from build123d import *

# Parameters (mm, degrees)
SALIENTE_EXTRUIR1_DEPTH = 3
SKETCH1_W               = 20
SKETCH1_H               = 7
SKETCH1_H_2             = 8
SKETCH1_W_2             = 7
SKETCH1_H_3             = 38.5
BOSS_EXTRUDE1_DEPTH     = 23
CUT_EXTRUDE1_DEPTH      = 85.65548432
SKETCH3_R               = 1.625
CUT_EXTRUDE2_DEPTH      = 73.427902257
SKETCH4_R               = 1
CUT_EXTRUDE3_DEPTH      = 4
CORTAR_EXTRUIR1_DEPTH   = 10
CORTAR_EXTRUIR2_REACH   = 71.098
CROQUIS4_R              = 1.25
CORTAR_EXTRUIR3_DEPTH   = 3
BOSS_EXTRUDE2_DEPTH     = 20
SALIENTE_EXTRUIR2_DEPTH = 10
CORTAR_EXTRUIR4_REACH   = 91.44
CROQUIS7_R              = 1.625
CORTAR_EXTRUIR5_START   = -6.425484
CORTAR_EXTRUIR5_DEPTH   = 4
SALIENTE_EXTRUIR3_DEPTH = 10
CORTAR_EXTRUIR6_REACH   = 91.44
CROQUIS10_R             = 1.625
CORTAR_EXTRUIR7_START   = -2.42548
CORTAR_EXTRUIR7_DEPTH   = 4


with BuildPart() as part:
    # Croquis1 → Saliente-Extruir1 (new body)
    with BuildSketch(Plane(origin=(0, 0, 0), x_dir=(1, 0, 0), z_dir=(0, 1, 0))):
        Polygon((-29.5, 32.640625), (29.5, 32.640625), (29.5, -47.359375), (8.5, -47.359375), (8.5, -27.453125), (3.5, -27.453125), (3.5, -47.359375), (-3.5, -47.359375), (-3.5, -27.453125), (-8.5, -27.453125), (-8.5, -47.359375), (-29.5, -47.359375), align=None)
    extrude(amount=SALIENTE_EXTRUIR1_DEPTH)

    # Sketch1 → Boss-Extrude1 (add)
    with BuildSketch(Plane(origin=(0, 3, 0), x_dir=(1, 0, 0), z_dir=(0, 1, 0))):
        with Locations((0, 19.640625)):
            Rectangle(SKETCH1_W, SKETCH1_H)
        with Locations((0, -12.359375)):
            Rectangle(SKETCH1_W, SKETCH1_H_2)
        with Locations((0, -35.609375)):
            Rectangle(SKETCH1_W_2, SKETCH1_H_3)
    extrude(amount=BOSS_EXTRUDE1_DEPTH)

    # Sketch2 → Cut-Extrude1 (cut, through all)
    with BuildSketch(Plane(origin=(29.5, 0, 0), x_dir=(0, 0, -1), z_dir=(1, 0, 0))):
        Polygon((-54.859375, 26), (-46.359375, 0), (-47.359375, 0), (-47.359375, 3), (-54.859375, 3), align=None)
    extrude(amount=-CUT_EXTRUDE1_DEPTH, mode=Mode.SUBTRACT)

    # Sketch3 → Cut-Extrude2 (cut, through all)
    with BuildSketch(Plane.ZY.offset(10)):
        with Locations((12.359375, 5.75)):
            Circle(SKETCH3_R)
        with Locations((12.359375, 23.25)):
            Circle(SKETCH3_R)
    extrude(amount=-CUT_EXTRUDE2_DEPTH, mode=Mode.SUBTRACT)

    # Sketch4 → Cut-Extrude3 (cut)
    with BuildSketch(Plane(origin=(0, -13.692511694, 41.882976946), x_dir=(1, 0, 0), z_dir=(0, -0.31073885630742226, 0.9504953251756452))):
        with Locations(Location((0, 19.405659167, 0), (0, 0, 270))):
            Circle(SKETCH4_R)
        with Locations(Location((0, 29.405659167, 0), (0, 0, 270))):
            Circle(SKETCH4_R)
    extrude(amount=-CUT_EXTRUDE3_DEPTH, mode=Mode.SUBTRACT)

    # Croquis2 → Cortar-Extruir1 (cut)
    with BuildSketch(Plane(origin=(0, 0, -23.140625), x_dir=(-1, 0, 0), z_dir=(0, 0, -1))):
        Polygon((-5, 6), (-5, 3), (5, 3), (5, 6), (5, 21), (-5, 21), align=None)
    extrude(amount=-CORTAR_EXTRUIR1_DEPTH, mode=Mode.SUBTRACT)

    # Croquis3 → Cortar-Extruir2 (cut, up to next)
    with BuildSketch(Plane.ZY.offset(3.5), mode=Mode.PRIVATE) as cortar_extruir2_sk1:
        Polygon((21.90625, 3), (36.90625, 3), (36.90625, 26), (21.90625, 26), (16.359375, 26), (16.359375, 3), align=None)
    cortar_extruir2_tool1 = extrude(cortar_extruir2_sk1.sketch, amount=-CORTAR_EXTRUIR2_REACH, mode=Mode.PRIVATE) & part.part
    add(cortar_extruir2_tool1.solids().sort_by_distance((-3.5, 14.5, 26.632812))[0], mode=Mode.SUBTRACT)

    # Croquis4 → Cortar-Extruir3 (cut)
    with BuildSketch(Plane.XZ):
        with Locations(Location((-24.5, -22.640625, 0), (0, 0, 270))):
            Circle(CROQUIS4_R)
        with Locations(Location((-16.5, -22.640625, 0), (0, 0, 270))):
            Circle(CROQUIS4_R)
        with Locations(Location((-16.5, -12.640625, 0), (0, 0, 270))):
            Circle(CROQUIS4_R)
        with Locations(Location((-16.5, -2.640625, 0), (0, 0, 270))):
            Circle(CROQUIS4_R)
        with Locations(Location((-16.5, 7.359375, 0), (0, 0, 270))):
            Circle(CROQUIS4_R)
        with Locations(Location((-16.5, 17.359375, 0), (0, 0, 270))):
            Circle(CROQUIS4_R)
        with Locations(Location((-16.5, 27.359375, 0), (0, 0, 270))):
            Circle(CROQUIS4_R)
        with Locations(Location((-16.5, 37.359375, 0), (0, 0, 270))):
            Circle(CROQUIS4_R)
        with Locations(Location((-24.5, -12.640625, 0), (0, 0, 270))):
            Circle(CROQUIS4_R)
        with Locations(Location((-24.5, -2.640625, 0), (0, 0, 270))):
            Circle(CROQUIS4_R)
        with Locations(Location((-24.5, 7.359375, 0), (0, 0, 270))):
            Circle(CROQUIS4_R)
        with Locations(Location((-24.5, 17.359375, 0), (0, 0, 270))):
            Circle(CROQUIS4_R)
        with Locations(Location((-24.5, 27.359375, 0), (0, 0, 270))):
            Circle(CROQUIS4_R)
        with Locations(Location((-24.5, 37.359375, 0), (0, 0, 270))):
            Circle(CROQUIS4_R)
        with Locations(Location((16.5, 37.359375, 0), (0, 0, 270))):
            Circle(CROQUIS4_R)
        with Locations(Location((24.5, 37.359375, 0), (0, 0, 270))):
            Circle(CROQUIS4_R)
        with Locations(Location((16.5, 27.359375, 0), (0, 0, 270))):
            Circle(CROQUIS4_R)
        with Locations(Location((24.5, 27.359375, 0), (0, 0, 270))):
            Circle(CROQUIS4_R)
        with Locations(Location((16.5, 17.359375, 0), (0, 0, 270))):
            Circle(CROQUIS4_R)
        with Locations(Location((24.5, 17.359375, 0), (0, 0, 270))):
            Circle(CROQUIS4_R)
        with Locations(Location((24.5, 7.359375, 0), (0, 0, 270))):
            Circle(CROQUIS4_R)
        with Locations(Location((16.5, 7.359375, 0), (0, 0, 270))):
            Circle(CROQUIS4_R)
        with Locations(Location((16.5, -2.640625, 0), (0, 0, 270))):
            Circle(CROQUIS4_R)
        with Locations(Location((24.5, -2.640625, 0), (0, 0, 270))):
            Circle(CROQUIS4_R)
        with Locations(Location((24.5, -12.640625, 0), (0, 0, 270))):
            Circle(CROQUIS4_R)
        with Locations(Location((16.5, -12.640625, 0), (0, 0, 270))):
            Circle(CROQUIS4_R)
        with Locations(Location((16.5, -22.640625, 0), (0, 0, 270))):
            Circle(CROQUIS4_R)
        with Locations(Location((24.5, -22.640625, 0), (0, 0, 270))):
            Circle(CROQUIS4_R)
        with Locations(Location((6, 22.084531493, 0), (0, 0, 270))):
            Circle(CROQUIS4_R)
        with Locations(Location((-6, 22.084531493, 0), (0, 0, 270))):
            Circle(CROQUIS4_R)
        with Locations(Location((6, 2.359375, 0), (0, 0, 270))):
            Circle(CROQUIS4_R)
        with Locations(Location((-6, 2.359375, 0), (0, 0, 270))):
            Circle(CROQUIS4_R)
        with Locations(Location((-6, -7.640625, 0), (0, 0, 270))):
            Circle(CROQUIS4_R)
        with Locations(Location((6, -7.640625, 0), (0, 0, 270))):
            Circle(CROQUIS4_R)
    extrude(amount=-CORTAR_EXTRUIR3_DEPTH, mode=Mode.SUBTRACT)

    # Sketch5 → Boss-Extrude2 (add)
    with BuildSketch(Plane(origin=(-8.5, 0, 0), x_dir=(0, 0, -1), z_dir=(1, 0, 0))):
        Polygon((-36.90625, 3), (-36.90625, 0), (-46.359375, 0), (-47.340144231, 3), align=None)
    extrude(amount=BOSS_EXTRUDE2_DEPTH)

    # Croquis6 → Saliente-Extruir2 (add)
    with BuildSketch(Plane.ZY.offset(29.5)):
        Polygon((44.340144231, 3), (47.340144231, 3), (50.447532794, 12.504953252), (44.340144231, 14.501599513), (44.340144231, 6.347956044), align=None)
        Polygon((40.990144231, 3), (44.340144231, 3), (44.340144231, 6.347956044), align=None)
    extrude(amount=-SALIENTE_EXTRUIR2_DEPTH)

    # Cortar-Extruir4: up to this plane
    cortar_extruir4_end = Plane(origin=(-19.5, 0, 44.340144231), z_dir=(0, 0, -1))
    # Croquis7 → Cortar-Extruir4 (cut, up to the surface)
    with BuildSketch(Plane(origin=(0, -13.692511694, 41.882976946), x_dir=(1, 0, 0), z_dir=(0, -0.31073885630742226, 0.9504953251756452)), mode=Mode.PRIVATE) as cortar_extruir4_sk1:
        with Locations(Location((-24.5, 22.561908251, 0), (0, 0, 270))):
            Circle(CROQUIS7_R)
    cortar_extruir4_tool1 = split(extrude(cortar_extruir4_sk1.sketch, amount=-CORTAR_EXTRUIR4_REACH, mode=Mode.PRIVATE), bisect_by=cortar_extruir4_end, keep=Keep.BOTH, mode=Mode.PRIVATE)
    add(cortar_extruir4_tool1.solids().sort_by_distance((-24.5, 7.752477, 48.893839))[0], mode=Mode.SUBTRACT)

    # Croquis8 → Cortar-Extruir5 (cut)
    with BuildSketch(Plane(origin=(0, -13.692511694, 41.882976946), x_dir=(1, 0, 0), z_dir=(0, -0.31073885630742226, 0.9504953251756452)).offset(CORTAR_EXTRUIR5_START)):
        Polygon((-22.91228676, 19.811908251), (-21.324573519, 22.561908251), (-22.91228676, 25.311908251), (-26.08771324, 25.311908251), (-27.675426481, 22.561908251), (-26.08771324, 19.811908251), align=None)
    extrude(amount=CORTAR_EXTRUIR5_DEPTH, mode=Mode.SUBTRACT)

    # Croquis9 → Saliente-Extruir3 (add)
    with BuildSketch(Plane(origin=(29.5, 0, 0), x_dir=(0, 0, -1), z_dir=(1, 0, 0))):
        Polygon((-50.447532794, 12.504953252), (-47.340144231, 3), (-44.340144231, 3), (-44.340144231, 6.347956044), (-44.340144231, 14.501599513), align=None)
        Polygon((-44.340144231, 6.347956044), (-44.340144231, 3), (-40.990144231, 3), align=None)
    extrude(amount=-SALIENTE_EXTRUIR3_DEPTH)

    # Cortar-Extruir6: up to this plane
    cortar_extruir6_end = Plane(origin=(19.5, 0, 44.340144231), z_dir=(0, 0, 1))
    # Croquis10 → Cortar-Extruir6 (cut, up to the surface)
    with BuildSketch(Plane(origin=(0, -13.692511694, 41.882976946), x_dir=(1, 0, 0), z_dir=(0, -0.31073885630742226, 0.9504953251756452)), mode=Mode.PRIVATE) as cortar_extruir6_sk1:
        with Locations(Location((24.5, 22.561908251, 0), (0, 0, 270))):
            Circle(CROQUIS10_R)
    cortar_extruir6_tool1 = split(extrude(cortar_extruir6_sk1.sketch, amount=-CORTAR_EXTRUIR6_REACH, mode=Mode.PRIVATE), bisect_by=cortar_extruir6_end, keep=Keep.BOTH, mode=Mode.PRIVATE)
    add(cortar_extruir6_tool1.solids().sort_by_distance((24.5, 7.752477, 48.893839))[0], mode=Mode.SUBTRACT)

    # Croquis11 → Cortar-Extruir7 (cut)
    with BuildSketch(Plane(origin=(0, -13.692511694, 41.882976946), x_dir=(1, 0, 0), z_dir=(0, -0.31073885630742226, 0.9504953251756452)).offset(CORTAR_EXTRUIR7_START)):
        Polygon((26.08771324, 19.811908251), (27.675426481, 22.561908251), (26.08771324, 25.311908251), (22.91228676, 25.311908251), (21.324573519, 22.561908251), (22.91228676, 19.811908251), align=None)
    extrude(amount=-CORTAR_EXTRUIR7_DEPTH, mode=Mode.SUBTRACT)


solid = part.part
Design review of the part built by this model. Coordinates are the model's own, in mm. A direction names the side the tool comes from. Round coordinates to 2 decimals unless told otherwise and drop trailing zeros. Write each loop counter-clockwise with the first axis right and the second up, starting at its lowest first coordinate (ties: lowest second). Pieces come first, ordered by that corner, then holes. Notation, with made-up numbers: M 76.5,68.25 L 87.5,68.25 A18 ccw 87.5,83.25 Z; hole C -10,-12 d7. An arc over 180 degrees is marked long. One line per item, written item: value. Start each with the question number.
1. To check wall thickness, follow probe 1 along Z at (x, y) = (7.5, 9); probe 2 along Z at (x, y) = (-4, 5.5); probe 3 along X at (y, z) = (12.5, 10.5). State the ranges of each line that lie inside material, in increasing order. Write a range as from..to.
2. Clearance check with flat-ended pins moving along their axes: P1, Ø3, axis at x = 16.5, z = 17.36, coming from the +Y side; P2, Ø2, axis at y = 15.5, z = -21, coming from the -X side; P3, Ø3, axis at x = -22.5, y = 6.5, coming from the +Z side; P4, Ø2, axis at x = 16.5, z = 7.36, coming from the +Y side. State where each tip first meets the part, or that it passes through.
3. Take a section at C-C on z = -12.5. State the section outline as (x, y) points.
4. For faces 1 (the face through (25, 13, 44.34)), 2 (the face through (-6, 2, 36.906)), 3 (the face through (-10, 14, 12)), 4 (the face through (-0.14, 5.821, 10.736)), 5 (the face through (-19.5, 9, 47)), list the 3-axis set-ups (+Z, -Z, +X, -X, +Y, -Y) from which the entire face can be reached by the end or side of a thin tool; tool diameter is ignored.
5. Take a section at B-B on y = 18. State the section outline as (x, z) points, then the cut area to 3 significant figures.
6. Draft analysis for pull direction Y (two halves, no side actions). For faces 6 (the face through (-24.57, 4.7, 42.69)), 7 (the face through (-24.478, 11.634, 45.87)), 8 (the face through (0, 1, -32.641)), 9 (the face through (0.3, 13.964, 48.85)), state which applies: pulls with the +Y half, pulls with the -Y half, needs draft (parallel to the pull), parting line crosses it, or undercut.
7. Take a section at A-A on x = -6. State how many separate pieces and enclosed holes the cut face has, then the cut area to 3 significant figures.
Computed:
1. probe 1: z = -23.14..-16.14, 8.36..16.36
1. probe 2: z = 8.36..10.75, 13.97..16.36
1. probe 3: x = -10..10
2. P1: stops at y = 3
2. P2: stops at x = -10
2. P3: stops at z = 48.97
2. P4: passes through
3. outline: M -29.5,0 L -25.74,0 L -25.74,3 L -29.5,3 Z; M -23.26,0 L -17.74,0 L -17.74,3 L -23.26,3 Z; M -15.26,0 L 15.26,0 L 15.26,3 L -15.26,3 Z; M 17.74,0 L 23.26,0 L 23.26,3 L 17.74,3 Z; M 25.74,0 L 29.5,0 L 29.5,3 L 25.74,3 Z
4. face 1: -Z, +X, +Y
4. face 2: +Y, -Y
4. face 3: +Z, -Z, -X, +Y
4. face 4: +X, -X
4. face 5: +Z, -Z, +Y
5. outline: M -10,-23.14 L -5,-23.14 L -5,-16.14 L -10,-16.14 Z; M -10,8.36 L 10,8.36 L 10,16.36 L -10,16.36 Z; M -3.5,36.91 L 3.5,36.91 L 3.5,52.24 L -3.5,52.24 Z; M 5,-23.14 L 10,-23.14 L 10,-16.14 L 5,-16.14 Z
5. area: 337 mm²
6. face 6: pulls with the +Y half
6. face 7: undercut
6. face 8: needs draft
6. face 9: undercut
7. separate pieces: 5
7. enclosed holes: 2
7. area: 516 mm²
